Here's how the part is built. I have some questions about the finished solid (model axes, mm). Face numbers are marked on the shaded views. Coordinates: 2 decimals unless noted, no trailing zeros. Write each loop counter-clockwise with the first axis right and the second up, starting at its lowest first coordinate (ties: lowest second). Pieces come first, ordered by that corner, then holes.
Item 1: If I drill on line 1 (X direction, y = 6.5, z = -17.5); line 2 (X direction, y = 4.75, z = 12); line 3 (Z direction, x = -24, y = 4.75), over which ranges is the centre line in solid material (lowest first)?
Item 2: If we section it at D-D (z = 20): Please give me the cut outline in (x, y).
Item 3: If we section it at B-B (y = 3.25): Please give me the cut outline in (x, z).
Item 4: If we section it at C-C (z = 28): Please give me the cut outline in (x, y).
Item 5: We'd pull the mould along Y, two halves only. Please class the marked faces 1 and 2: +Y half, -Y half, draft (parallel to the pull), parting line (faces both ways), or undercut.
Item 6: If we section it at A-A (x = 10): Please give me the cut outline in (y, z).
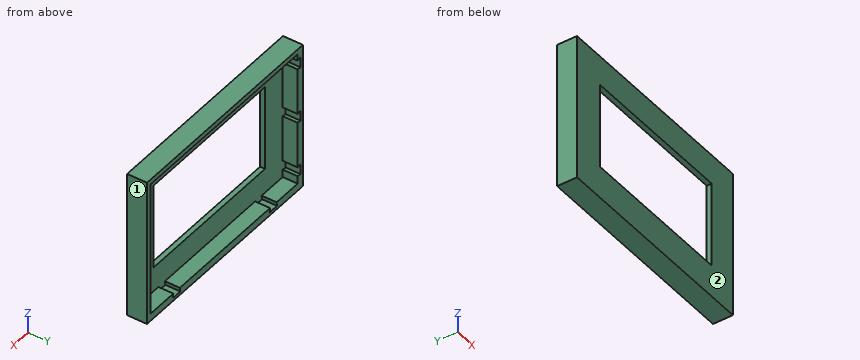
from build123d import *

# Parameters (mm, degrees)
SKETCH1_W           = 88.3
SKETCH1_H           = 59.5
BOSS_EXTRUDE1_DEPTH = 8
SKETCH2_W           = 83.3
SKETCH2_H           = 54.5
CUT_EXTRUDE1_DEPTH  = 6
CUT_EXTRUDE2_DEPTH  = 6
SKETCH4_W           = 63.3
SKETCH4_H           = 34.5
CUT_EXTRUDE3_DEPTH  = 3


with BuildPart() as part:
    # Sketch1 → Boss-Extrude1 (new body)
    with BuildSketch(Plane(origin=(0, 0, 0), x_dir=(1, 0, 0), z_dir=(0, 1, 0))):
        with Locations((5.926671878, -4.296406043)):
            Rectangle(SKETCH1_W, SKETCH1_H)
    extrude(amount=BOSS_EXTRUDE1_DEPTH)

    # Sketch2 → Cut-Extrude1 (cut)
    with BuildSketch(Plane(origin=(0, 8, 0), x_dir=(1, 0, 0), z_dir=(0, 1, 0))):
        with Locations((6.426671878, -4.796406043)):
            Rectangle(SKETCH2_W, SKETCH2_H)
    extrude(amount=-CUT_EXTRUDE1_DEPTH, mode=Mode.SUBTRACT)

    # Sketch3 → Cut-Extrude2 (cut)
    with BuildSketch(Plane(origin=(0, 8, 0), x_dir=(1, 0, 0), z_dir=(0, 1, 0))):
        Polygon((-35.223328122, -29.396406043), (-36.923328122, -29.646406043), (-36.923328122, -25.446406043), (-35.223328122, -25.696406043), align=None)
        Polygon((-35.223328122, -6.896406043), (-36.923328122, -7.146406043), (-36.923328122, -2.946406043), (-35.223328122, -3.196406043), align=None)
        Polygon((-35.223328122, 15.603593957), (-36.923328122, 15.353593957), (-36.923328122, 19.553593957), (-35.223328122, 19.303593957), align=None)
        Polygon((35.176671878, 22.453593957), (31.476671878, 22.453593957), (31.226671878, 24.153593957), (35.426671878, 24.153593957), align=None)
        Polygon((-23.323328122, 22.453593957), (-23.573328122, 24.153593957), (-19.373328122, 24.153593957), (-19.623328122, 22.453593957), align=None)
    extrude(amount=-CUT_EXTRUDE2_DEPTH, mode=Mode.SUBTRACT)

    # Sketch4 → Cut-Extrude3 (cut, through all)
    with BuildSketch(Plane(origin=(0, 2, 0), x_dir=(1, 0, 0), z_dir=(0, 1, 0))):
        with Locations((6.426671878, -4.796406043)):
            Rectangle(SKETCH4_W, SKETCH4_H)
    extrude(amount=-CUT_EXTRUDE3_DEPTH, mode=Mode.SUBTRACT)


solid = part.part
Answer list:
1. line 1: x = -38.22 to -36.92, 48.08 to 50.08
1. line 2: x = -38.22 to -35.22, 48.08 to 50.08
1. line 3: z = -25.45 to -22.45, 32.05 to 34.05
2. outline: (-38.22, 0) - (-25.22, 0) - (-25.22, 2) - (-35.22, 2) - (-35.22, 8) - (-38.22, 8) - close; (38.08, 0) - (50.08, 0) - (50.08, 8) - (48.08, 8) - (48.08, 2) - (38.08, 2) - close
3. outline: (-38.22, -25.45) - (50.08, -25.45) - (50.08, 34.05) - (-38.22, 34.05) - close; hole (-36.92, -19.55) - (-35.22, -19.3) - (-35.22, -22.45) - (-23.32, -22.45) - (-23.57, -24.15) - (-19.37, -24.15) - (-19.62, -22.45) - (31.48, -22.45) - (31.23, -24.15) - (35.43, -24.15) - (35.18, -22.45) - (48.08, -22.45) - (48.08, 32.05) - (-35.22, 32.05) - (-35.22, 29.4) - (-36.92, 29.65) - (-36.92, 25.45) - (-35.22, 25.7) - (-35.22, 6.9) - (-36.92, 7.15) - (-36.92, 2.95) - (-35.22, 3.2) - (-35.22, -15.6) - (-36.92, -15.35) - close
4. outline: (-38.22, 0) - (50.08, 0) - (50.08, 8) - (48.08, 8) - (48.08, 2) - (-36.92, 2) - (-36.92, 8) - (-38.22, 8) - close
5. face 1: draft
5. face 2: -Y half
6. outline: (0, -25.45) - (8, -25.45) - (8, -22.45) - (2, -22.45) - (2, -12.45) - (0, -12.45) - close; (0, 22.05) - (2, 22.05) - (2, 32.05) - (8, 32.05) - (8, 34.05) - (0, 34.05) - close
